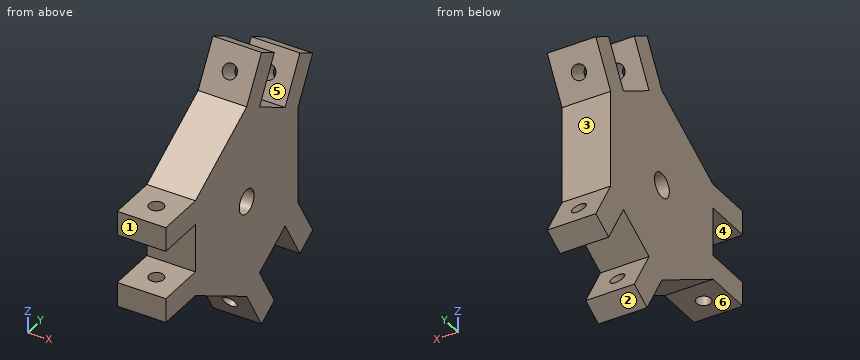
```python
from build123d import *

# Parameters (mm, degrees)
EXTRUDE_1_DEPTH          = 20
SKETCH_2_W               = 20
SKETCH_2_H               = 10
EXTRUDE_2_DEPTH          = 20
SKETCH_3_W               = 20
SKETCH_3_H               = 10
EXTRUDE_3_DEPTH          = 20
SKETCH_4_R               = 3
CUT_EXTRUDE_1_DEPTH      = 88.361609461
CUT_EXTRUDE_2_DEPTH      = 76.355563624
CUT_EXTRUDE_2_DEPTH_BACK = 76.355563624
SKETCH_5_R               = 5
PATTERN_CIRCULAR_1_COUNT = 3


with BuildPart() as part:
    # 草图1 → 凸台-拉伸1 (new body)
    with BuildSketch(Plane(origin=(0, 0, 0), x_dir=(0, 0, -1), z_dir=(1, 0, 0))):
        Polygon((20, -34.641016151), (-20, -34.641016151), (-40, 0), (-20, 34.641016151), (20, 34.641016151), (40, 0), align=None)
    extrude(amount=EXTRUDE_1_DEPTH)

    # 草图2 → 凸台-拉伸2 (add)
    with BuildSketch(Plane(origin=(0, 17.320508076, 30), x_dir=(1, 0, 0), z_dir=(0, 0.500000000000003, 0.8660254037844369))):
        with Locations((10, 15)):
            Rectangle(SKETCH_2_W, SKETCH_2_H)
    extrude_2 = extrude(amount=EXTRUDE_2_DEPTH)

    # 草图3 → 凸台-拉伸3 (add)
    with BuildSketch(Plane(origin=(0, 17.320508076, 30), x_dir=(1, 0, 0), z_dir=(0, 0.500000000000003, 0.8660254037844369))):
        with Locations((10, -15)):
            Rectangle(SKETCH_3_W, SKETCH_3_H)
    extrude_3 = extrude(amount=EXTRUDE_3_DEPTH)

    # 草图4 → 切除-拉伸1 (cut, symmetric)
    with BuildSketch(Plane(origin=(0, 17.320508076, -10), x_dir=(1, 0, 0), z_dir=(0, 0.8660254037844369, -0.500000000000003))):
        with Locations(Location((10, -44.641016151, 0), (0, 0, 270))):
            Circle(SKETCH_4_R)
    cut_extrude_1 = extrude(amount=CUT_EXTRUDE_1_DEPTH, both=True, mode=Mode.SUBTRACT)

    # 草图5 → 切除-拉伸2 (cut, two sides: drawn at the far end of the back side and taken through both)
    with BuildSketch(Plane(origin=(20, 0, 0), x_dir=(0, 0, -1), z_dir=(1, 0, 0)).offset(-CUT_EXTRUDE_2_DEPTH_BACK)):
        Circle(SKETCH_5_R)
    extrude(amount=CUT_EXTRUDE_2_DEPTH + CUT_EXTRUDE_2_DEPTH_BACK, mode=Mode.SUBTRACT)

    # 阵列(圆周)1: 凸台-拉伸2, 凸台-拉伸3, 切除-拉伸1 ×3 about axis
    pattern_circular_1_axis = Axis((0, 0, 0), (1, 0, 0))
    add([extrude_2.rotate(pattern_circular_1_axis, i * 360 / PATTERN_CIRCULAR_1_COUNT) for i in range(1, PATTERN_CIRCULAR_1_COUNT)])
    add([extrude_3.rotate(pattern_circular_1_axis, i * 360 / PATTERN_CIRCULAR_1_COUNT) for i in range(1, PATTERN_CIRCULAR_1_COUNT)])
    add([cut_extrude_1.rotate(pattern_circular_1_axis, i * 360 / PATTERN_CIRCULAR_1_COUNT) for i in range(1, PATTERN_CIRCULAR_1_COUNT)], mode=Mode.SUBTRACT)


solid = part.part
```
The model under review builds one solid part; all positions refer to its coordinate system, in mm. Face numbers are marked on the shaded views. A direction names the side the tool comes from. Round coordinates to 2 decimals unless told otherwise and drop trailing zeros. Loops run counter-clockwise (first coordinate to the right, second up) from the corner with the lowest first, then second, coordinate; pieces in that order, holes last. Notation, with made-up numbers: (18.25, 80) -> (54.25, 80) arc R6 cw to (54.25, 85) -> close; hole circle Ø5 at (42, 16.25). An arc over 180 degrees is marked (long way). Answer as a JSON object with one key per item and string values. Group by question number.
1) Mouldability with a two-part tool opening along Z and no side actions: class the marked faces 1, 2 and 3 as released by +Z, released by -Z, zero draft, split by the parting line, or undercut.
2) For line 1 (Y direction, x = 7, z = 0); line 2 (Z direction, x = 8.25, y = -48.5); line 3 (Z direction, x = 11.5, y = 13), list the stretches that pass through material, from the lowest coordinate up. Write a range as [from, to].
3) For the marked faces 4, 5 and 6, list the 3-axis set-ups (+Z, -Z, +X, -X, +Y, -Y) from which the entire face can be reached by the end or side of a thin tool; tool diameter is ignored.
4) We need section D-D on x = 3.25. Write out the cut boundary in (y, z), then the cut area to 3 significant figures.
5) We need section B-B on y = 17. Write out the cut boundary in (x, z), then the cut area to 3 significant figures.
6) We need section C-C on z = 15.5. Write out the cut boundary in (x, y).
7) We need section A-A on z = 0. Write out the cut boundary in (x, y).
8) For pin 1 Ø10 at (x, y) = (16, -10) entering from +Z; pin 2 Ø5 at (x, y) = (10, -44.64) entering from -Z; pin 3 Ø6 at (x, y) = (12, -45.5) entering from -Z; pin 4 Ø10 at (x, z) = (3, 23.5) entering from +Y, all flat-tipped, find the tip position at first contact; note any pin that passes through.
Result set:
{
 "1": {"face 1": "zero draft", "face 2": "released by -Z", "face 3": "undercut"},
 "2": {"line 1": "[-34.64, -5], [5, 34.64]", "line 2": "[-20, -10], [10, 20]", "line 3": "[-55.59, -47.04], [-32.49, 32.49], [47.04, 55.59]"},
 "3": {"face 4": "+X, -X, -Y", "face 5": "+Z, +X, -X", "face 6": "-Z, +X, -X, -Y"},
 "4": {"outline": "(-54.64, -20) -> (-34.64, -20) -> (0, -40) -> (10, -57.32) -> (18.66, -52.32) -> (8.66, -35) -> (25.98, -25) -> (35.98, -42.32) -> (44.64, -37.32) -> (34.64, -20) -> (34.64, 20) -> (44.64, 37.32) -> (35.98, 42.32) -> (25.98, 25) -> (8.66, 35) -> (18.66, 52.32) -> (10, 57.32) -> (0, 40) -> (-34.64, 20) -> (-54.64, 20) -> (-54.64, 10) -> (-34.64, 10) -> (-34.64, -10) -> (-54.64, -10) -> close; hole circle Ø10 at (0, 0)", "area": "5,280 mm²"},
 "5": {"outline": "(0, -53.28) -> (20, -53.28) -> (20, -49.44) -> (0, -49.44) -> close; (0, -30.19) -> (20, -30.19) -> (20, 30.19) -> (0, 30.19) -> close; (0, 49.44) -> (20, 49.44) -> (20, 53.28) -> (0, 53.28) -> close", "area": "1,360 mm²"},
 "6": {"outline": "(0, -54.64) -> (20, -54.64) -> (20, 34.64) -> (0, 34.64) -> close; hole circle Ø6 at (10, -44.64)"},
 "7": {"outline": "(0, -34.64) -> (20, -34.64) -> (20, -5) -> (0, -5) -> close; (0, 5) -> (20, 5) -> (20, 34.64) -> (0, 34.64) -> close"},
 "8": {"pin 1": "z = 37.11", "pin 2": "through", "pin 3": "z = -20", "pin 4": "y = 39.55"}
}
